Read the model definition and answer for the solid it produces. Units are mm, in the model's axes. Face numbers are marked on the shaded views. A direction names the side the tool comes from. Give positions to 0.01 mm unless a question says otherwise; leave off trailing zeros. Write each loop counter-clockwise with the first axis right and the second up, starting at its lowest first coordinate (ties: lowest second). Pieces come first, ordered by that corner, then holes. Notation, with made-up numbers: M 48,85.5 L 64,85.5 A18 ccw 64,92.5 Z; hole C 35,37.5 d10. An arc over 180 degrees is marked long. Put each result on its own line as item: value.
from build123d import *

# Parameters (mm, degrees)
SKETCH1_W               = 228.6
SKETCH1_H               = 228.6
BOSS_EXTRUDE1_DEPTH     = 140
SKETCH2_W               = 35.766
SKETCH2_H               = 35.766
CUT_EXTRUDE1_DEPTH      = 76.2
CUT_EXTRUDE3_DEPTH      = 4
CUT_EXTRUDE3_DEPTH_BACK = 4
SKETCH4_W               = 140
SKETCH4_H               = 35.766
CUT_EXTRUDE4_DEPTH      = 4
CUT_EXTRUDE4_DEPTH_BACK = 4
SKETCH5_W               = 140
SKETCH5_H               = 37.77
SKETCH5_H_2             = 35.766
CUT_EXTRUDE5_DEPTH      = 4
CUT_EXTRUDE5_DEPTH_BACK = 4
SKETCH6_W               = 140
SKETCH6_H               = 35.766
SKETCH6_H_2             = 37.77
CUT_EXTRUDE6_DEPTH      = 4
CUT_EXTRUDE6_DEPTH_BACK = 4
SKETCH9_W               = 140
SKETCH9_H               = 37.766
SKETCH9_H_2             = 35.766
SKETCH9_H_3             = 37.77
SKETCH10_W              = 140
SKETCH10_H              = 2
CUT_EXTRUDE7_DEPTH      = 263.834749521
SKETCH11_W              = 140
SKETCH11_H              = 2
CUT_EXTRUDE8_DEPTH      = 262.383356203
SKETCH12_W              = 33.77
SKETCH12_H              = 33.766
SKETCH12_W_2            = 35.766
SKETCH12_W_3            = 33.766
SKETCH12_H_2            = 35.766
SKETCH12_H_3            = 33.77
CUT_EXTRUDE9_DEPTH      = 177.150560601
SKETCH13_W              = 33.77
SKETCH13_H              = 35.766
SKETCH13_W_2            = 35.766
CUT_EXTRUDE10_DEPTH     = 177.150560601
SKETCH14_W              = 35.766
SKETCH14_H              = 35.766
CUT_EXTRUDE11_DEPTH     = 177.150560601


with BuildPart() as part:
    # Sketch1 → Boss-Extrude1 (new body)
    with BuildSketch(Plane(origin=(0, 0, 0), x_dir=(0, 0, -1), z_dir=(1, 0, 0))):
        Rectangle(SKETCH1_W, SKETCH1_H)
    extrude(amount=BOSS_EXTRUDE1_DEPTH)

    # Sketch2 → Cut-Extrude1 (cut)
    with BuildSketch(Plane(origin=(140, 0, 0), x_dir=(0, 0, -1), z_dir=(1, 0, 0))):
        with Locations((-94.417, 94.417)):
            Rectangle(SKETCH2_W, SKETCH2_H)
        with Locations((-56.651, 94.417)):
            Rectangle(SKETCH2_W, SKETCH2_H)
        with Locations((18.881, 94.417)):
            Rectangle(SKETCH2_W, SKETCH2_H)
        with Locations((-18.885, 94.417)):
            Rectangle(SKETCH2_W, SKETCH2_H)
        with Locations((56.647, 94.417)):
            Rectangle(SKETCH2_W, SKETCH2_H)
        with Locations((94.413, 94.417)):
            Rectangle(SKETCH2_W, SKETCH2_H)
        with Locations((56.647, 56.651)):
            Rectangle(SKETCH2_W, SKETCH2_H)
        with Locations((94.413, 56.651)):
            Rectangle(SKETCH2_W, SKETCH2_H)
        with Locations((18.881, 56.651)):
            Rectangle(SKETCH2_W, SKETCH2_H)
        with Locations((-18.885, 56.651)):
            Rectangle(SKETCH2_W, SKETCH2_H)
        with Locations((-56.651, 56.651)):
            Rectangle(SKETCH2_W, SKETCH2_H)
        with Locations((-94.417, 56.651)):
            Rectangle(SKETCH2_W, SKETCH2_H)
        with Locations((-94.417, 18.885)):
            Rectangle(SKETCH2_W, SKETCH2_H)
        with Locations((-56.651, 18.885)):
            Rectangle(SKETCH2_W, SKETCH2_H)
        with Locations((-18.885, 18.885)):
            Rectangle(SKETCH2_W, SKETCH2_H)
        with Locations((18.881, 18.885)):
            Rectangle(SKETCH2_W, SKETCH2_H)
        with Locations((56.647, 18.885)):
            Rectangle(SKETCH2_W, SKETCH2_H)
        with Locations((94.413, 18.885)):
            Rectangle(SKETCH2_W, SKETCH2_H)
        with Locations((94.413, -18.881)):
            Rectangle(SKETCH2_W, SKETCH2_H)
        with Locations((56.647, -18.881)):
            Rectangle(SKETCH2_W, SKETCH2_H)
        with Locations((18.881, -18.881)):
            Rectangle(SKETCH2_W, SKETCH2_H)
        with Locations((-18.885, -18.881)):
            Rectangle(SKETCH2_W, SKETCH2_H)
        with Locations((-56.651, -18.881)):
            Rectangle(SKETCH2_W, SKETCH2_H)
        with Locations((-94.417, -18.881)):
            Rectangle(SKETCH2_W, SKETCH2_H)
        with Locations((56.647, -56.647)):
            Rectangle(SKETCH2_W, SKETCH2_H)
        with Locations((94.413, -56.647)):
            Rectangle(SKETCH2_W, SKETCH2_H)
        with Locations((94.413, -94.413)):
            Rectangle(SKETCH2_W, SKETCH2_H)
        with Locations((56.647, -94.413)):
            Rectangle(SKETCH2_W, SKETCH2_H)
        with Locations((18.881, -94.413)):
            Rectangle(SKETCH2_W, SKETCH2_H)
        with Locations((18.881, -56.647)):
            Rectangle(SKETCH2_W, SKETCH2_H)
        with Locations((-18.885, -56.647)):
            Rectangle(SKETCH2_W, SKETCH2_H)
        with Locations((-18.885, -94.413)):
            Rectangle(SKETCH2_W, SKETCH2_H)
        with Locations((-56.651, -94.413)):
            Rectangle(SKETCH2_W, SKETCH2_H)
        with Locations((-56.651, -56.647)):
            Rectangle(SKETCH2_W, SKETCH2_H)
        with Locations((-94.417, -94.413)):
            Rectangle(SKETCH2_W, SKETCH2_H)
        with Locations((-94.417, -56.647)):
            Rectangle(SKETCH2_W, SKETCH2_H)
    extrude(amount=-CUT_EXTRUDE1_DEPTH, mode=Mode.SUBTRACT)

    # Sketch4 → Cut-Extrude3 (cut, two sides: drawn at the far end of the back side and taken through both)
    with BuildSketch(Plane(origin=(0, -114.3, 0), x_dir=(1, 0, 0), z_dir=(0, 1, 0)).offset(-CUT_EXTRUDE3_DEPTH_BACK)):
        with Locations((70, -94.417)):
            Rectangle(SKETCH4_W, SKETCH4_H)
        with Locations((70, -56.651)):
            Rectangle(SKETCH4_W, SKETCH4_H)
        with Locations((70, -18.885)):
            Rectangle(SKETCH4_W, SKETCH4_H)
        with Locations((70, 18.881)):
            Rectangle(SKETCH4_W, SKETCH4_H)
        with Locations((70, 56.647)):
            Rectangle(SKETCH4_W, SKETCH4_H)
        with Locations((70, 94.413)):
            Rectangle(SKETCH4_W, SKETCH4_H)
    extrude(amount=CUT_EXTRUDE3_DEPTH + CUT_EXTRUDE3_DEPTH_BACK, mode=Mode.SUBTRACT)

    # Sketch5 → Cut-Extrude4 (cut, two sides: drawn at the far end of the back side and taken through both)
    with BuildSketch(Plane.XY.offset(114.3).offset(-CUT_EXTRUDE4_DEPTH_BACK)):
        with Locations((70, -95.415)):
            Rectangle(SKETCH5_W, SKETCH5_H)
        with Locations((70, -56.647)):
            Rectangle(SKETCH5_W, SKETCH5_H_2)
        with Locations((70, -18.881)):
            Rectangle(SKETCH5_W, SKETCH5_H_2)
        with Locations((70, 18.885)):
            Rectangle(SKETCH5_W, SKETCH5_H_2)
        with Locations((70, 56.651)):
            Rectangle(SKETCH5_W, SKETCH5_H_2)
        with Locations((70, 94.417)):
            Rectangle(SKETCH5_W, SKETCH5_H_2)
    extrude(amount=CUT_EXTRUDE4_DEPTH + CUT_EXTRUDE4_DEPTH_BACK, mode=Mode.SUBTRACT)

    # Sketch6 → Cut-Extrude5 (cut, two sides: drawn at the far end of the back side and taken through both)
    with BuildSketch(Plane.XY.offset(-114.3).offset(-CUT_EXTRUDE5_DEPTH_BACK)):
        with Locations((70, 94.417)):
            Rectangle(SKETCH6_W, SKETCH6_H)
        with Locations((70, 56.651)):
            Rectangle(SKETCH6_W, SKETCH6_H)
        with Locations((70, 18.885)):
            Rectangle(SKETCH6_W, SKETCH6_H)
        with Locations((70, -18.881)):
            Rectangle(SKETCH6_W, SKETCH6_H)
        with Locations((70, -56.647)):
            Rectangle(SKETCH6_W, SKETCH6_H)
        with Locations((70, -95.415)):
            Rectangle(SKETCH6_W, SKETCH6_H_2)
    extrude(amount=CUT_EXTRUDE5_DEPTH + CUT_EXTRUDE5_DEPTH_BACK, mode=Mode.SUBTRACT)

    # Sketch9 → Cut-Extrude6 (cut, two sides: drawn at the far end of the back side and taken through both)
    with BuildSketch(Plane(origin=(0, 114.3, 0), x_dir=(1, 0, 0), z_dir=(0, 1, 0)).offset(-CUT_EXTRUDE6_DEPTH_BACK)):
        with Locations((70, -95.417)):
            Rectangle(SKETCH9_W, SKETCH9_H)
        with Locations((70, -56.651)):
            Rectangle(SKETCH9_W, SKETCH9_H_2)
        with Locations((70, -18.885)):
            Rectangle(SKETCH9_W, SKETCH9_H_2)
        with Locations((70, 18.881)):
            Rectangle(SKETCH9_W, SKETCH9_H_2)
        with Locations((70, 56.647)):
            Rectangle(SKETCH9_W, SKETCH9_H_2)
        with Locations((70, 95.415)):
            Rectangle(SKETCH9_W, SKETCH9_H_3)
    extrude(amount=CUT_EXTRUDE6_DEPTH + CUT_EXTRUDE6_DEPTH_BACK, mode=Mode.SUBTRACT)

    # Sketch10 → Cut-Extrude7 (cut, through all)
    with BuildSketch(Plane.XY.offset(76.534)):
        with Locations((70, -113.3)):
            Rectangle(SKETCH10_W, SKETCH10_H)
        with Locations((70, 113.3)):
            Rectangle(SKETCH10_W, SKETCH10_H)
    extrude(amount=-CUT_EXTRUDE7_DEPTH, mode=Mode.SUBTRACT)

    # Sketch11 → Cut-Extrude8 (cut, through all)
    with BuildSketch(Plane(origin=(0, -76.53, 0), x_dir=(-1, 0, 0), z_dir=(0, -1, 0))):
        with Locations((-70, 113.3)):
            Rectangle(SKETCH11_W, SKETCH11_H)
        with Locations((-70, -113.3)):
            Rectangle(SKETCH11_W, SKETCH11_H)
    extrude(amount=-CUT_EXTRUDE8_DEPTH, mode=Mode.SUBTRACT)

    # Sketch12 → Cut-Extrude9 (cut, through all)
    with BuildSketch(Plane(origin=(63.8, 0, 0), x_dir=(0, 0, -1), z_dir=(1, 0, 0))):
        with Locations((93.415, 93.417)):
            Rectangle(SKETCH12_W, SKETCH12_H)
        with Locations((56.647, 93.417)):
            Rectangle(SKETCH12_W_2, SKETCH12_H)
        with Locations((-18.885, 93.417)):
            Rectangle(SKETCH12_W_2, SKETCH12_H)
        with Locations((18.881, 93.417)):
            Rectangle(SKETCH12_W_2, SKETCH12_H)
        with Locations((-56.651, 93.417)):
            Rectangle(SKETCH12_W_2, SKETCH12_H)
        with Locations((-93.417, 93.417)):
            Rectangle(SKETCH12_W_3, SKETCH12_H)
        with Locations((-93.417, 56.651)):
            Rectangle(SKETCH12_W_3, SKETCH12_H_2)
        with Locations((-93.417, 18.885)):
            Rectangle(SKETCH12_W_3, SKETCH12_H_2)
        with Locations((-93.417, -18.881)):
            Rectangle(SKETCH12_W_3, SKETCH12_H_2)
        with Locations((-93.417, -56.647)):
            Rectangle(SKETCH12_W_3, SKETCH12_H_2)
        with Locations((-93.417, -93.415)):
            Rectangle(SKETCH12_W_3, SKETCH12_H_3)
        with Locations((-56.651, -93.415)):
            Rectangle(SKETCH12_W_2, SKETCH12_H_3)
        with Locations((-18.885, -93.415)):
            Rectangle(SKETCH12_W_2, SKETCH12_H_3)
        with Locations((18.881, -93.415)):
            Rectangle(SKETCH12_W_2, SKETCH12_H_3)
        with Locations((56.647, -93.415)):
            Rectangle(SKETCH12_W_2, SKETCH12_H_3)
        with Locations((93.415, -93.415)):
            Rectangle(SKETCH12_W, SKETCH12_H_3)
        with Locations((93.415, -56.647)):
            Rectangle(SKETCH12_W, SKETCH12_H_2)
        with Locations((93.415, -18.881)):
            Rectangle(SKETCH12_W, SKETCH12_H_2)
    extrude(amount=-CUT_EXTRUDE9_DEPTH, mode=Mode.SUBTRACT)

    # Sketch13 → Cut-Extrude10 (cut, through all)
    with BuildSketch(Plane(origin=(63.8, 0, 0), x_dir=(0, 0, -1), z_dir=(1, 0, 0))):
        with Locations((93.415, 18.885)):
            Rectangle(SKETCH13_W, SKETCH13_H)
        with Locations((93.415, 56.651)):
            Rectangle(SKETCH13_W, SKETCH13_H)
        with Locations((56.647, 56.651)):
            Rectangle(SKETCH13_W_2, SKETCH13_H)
        with Locations((18.881, 56.651)):
            Rectangle(SKETCH13_W_2, SKETCH13_H)
        with Locations((18.881, 18.885)):
            Rectangle(SKETCH13_W_2, SKETCH13_H)
        with Locations((56.647, 18.885)):
            Rectangle(SKETCH13_W_2, SKETCH13_H)
        with Locations((-18.885, 18.885)):
            Rectangle(SKETCH13_W_2, SKETCH13_H)
        with Locations((-56.651, 18.885)):
            Rectangle(SKETCH13_W_2, SKETCH13_H)
        with Locations((-56.651, -18.881)):
            Rectangle(SKETCH13_W_2, SKETCH13_H)
        with Locations((-56.651, -56.647)):
            Rectangle(SKETCH13_W_2, SKETCH13_H)
        with Locations((18.881, -56.647)):
            Rectangle(SKETCH13_W_2, SKETCH13_H)
        with Locations((-18.885, -56.647)):
            Rectangle(SKETCH13_W_2, SKETCH13_H)
        with Locations((56.647, -56.647)):
            Rectangle(SKETCH13_W_2, SKETCH13_H)
        with Locations((56.647, -18.881)):
            Rectangle(SKETCH13_W_2, SKETCH13_H)
    extrude(amount=-CUT_EXTRUDE10_DEPTH, mode=Mode.SUBTRACT)

    # Sketch14 → Cut-Extrude11 (cut, through all)
    with BuildSketch(Plane(origin=(63.8, 0, 0), x_dir=(0, 0, -1), z_dir=(1, 0, 0))):
        with Locations((18.881, -18.881)):
            Rectangle(SKETCH14_W, SKETCH14_H)
        with Locations((-18.885, -18.881)):
            Rectangle(SKETCH14_W, SKETCH14_H)
        with Locations((-18.885, 56.651)):
            Rectangle(SKETCH14_W, SKETCH14_H)
        with Locations((-56.651, 56.651)):
            Rectangle(SKETCH14_W, SKETCH14_H)
    extrude(amount=-CUT_EXTRUDE11_DEPTH, mode=Mode.SUBTRACT)


solid = part.part
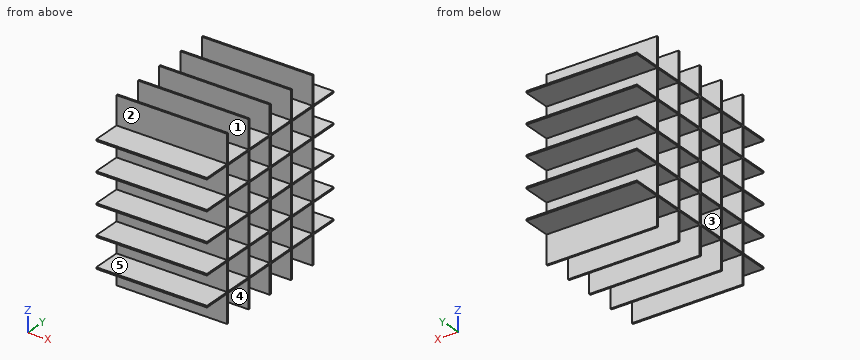
(1) Section A-A on y = 99.5 is taken. Determine the outline of the cut face in (x, z).
Result:
outline: M 0,-76.53 L 140,-76.53 L 140,-74.53 L 0,-74.53 Z; M 0,-38.76 L 140,-38.76 L 140,-36.76 L 0,-36.76 Z; M 0,-1 L 140,-1 L 140,1 L 0,1 Z; M 0,36.77 L 140,36.77 L 140,38.77 L 0,38.77 Z; M 0,74.53 L 140,74.53 L 140,76.53 L 0,76.53 Z
(2) Given pin 1 Ø10.5 at (x, y) = (96.5, -90.5) entering from +Z; pin 2 Ø1.5 at (x, y) = (81.5, -66) entering from -Z; pin 3 Ø18 at (x, z) = (39, 22.5) entering from -Y; pin 4 Ø8 at (y, z) = (84.5, 53.5) entering from +X, each flat-ended and moving along its own axis, determine where each tip first touches the part or whether it passes through.
Result:
pin 1: stops at z = 76.53
pin 2: stops at z = -76.53
pin 3: stops at y = -76.53
pin 4: passes through
(3) A straight line is drawn through the part: line 1 along Z through (x, y) = (57, -30.5). Find the intervals that lie inside material, in ascending order. Write a range as from..to.
Result:
line 1: z = -76.53..-74.53, -38.76..-36.76, -1..1, 36.77..38.77, 74.53..76.53
(4) Section C-C on x = 92.5 is taken. Give the number of separate pieces and of enclosed holes in the cut face, and give its area (3 significant figures).
Result:
separate pieces: 1
enclosed holes: 16
area: 4,390 mm²
(5) Which of the six approach directions +Z, -Z, +X, -X, +Y, -Y give full straight-line access (tool end or side, diameter ignored) to the marked faces 1, 2, 3, 4 and 5?
Result:
face 1: +Z, +X, -X
face 2: +Z, +X, -X, -Y
face 3: +X, -X
face 4: -Z, +X, -X
face 5: +X, -X, -Y
